For this review, use the dimensioned drawing (mm, ordinates from the lowest corner) and the shaded views. A direction names the side the tool comes from. Round coordinates to 2 decimals unless told otherwise and drop trailing zeros. Write each loop counter-clockwise with the first axis right and the second up, starting at its lowest first coordinate (ties: lowest second). Pieces come first, ordered by that corner, then holes. Notation, with made-up numbers: M -16.75,27.25 L 31.25,27.25 A19 cw 31.25,36.25 Z; hole C 76,-1.5 d7. An arc over 180 degrees is marked long. Use one line per item in the form item = value. Start each with the question number.
Item 1: Add section B-B (z = 2). State the section outline as (x, y) points.
Item 2: For the marked faces 1, 2, 3, 4 and 5, list the 3-axis set-ups (+Z, -Z, +X, -X, +Y, -Y) from which the entire face can be reached by the end or side of a thin tool; tool diameter is ignored.
Item 3: Draft analysis for pull direction X (two halves, no side actions). For the marked faces 6, 7 and 8, state which applies: released by +X, released by -X, zero draft, split by the parting line, or undercut.
Item 4: For P1, Ø1.2, axis at y = 12, z = 5, coming from the -X side; P2, Ø2, axis at x = 5.5, z = 4, coming from the +Y side; P3, Ø4, axis at x = 1.5, z = 5, coming from the -Y side; P4, Ø3, axis at y = 2.5, z = 6.5, coming from the +X side, all flat-tipped, find the tip position at first contact; note any pin that passes through.
Item 5: Add section D-D (z = 4.25). Count the separate pieces of the cut face and the enclosed holes in it, and give its area (3 significant figures).
Item 6: For line 1 (X direction, y = 13.25, z = 5); line 2 (Y direction, x = 5, z = 3.6); line 3 (Z direction, x = 1.95, y = 12), list the stretches that pass through material, from the lowest coordinate up. Write a range as [from, to].
Item 7: Add section A-A (y = 9.5). State the section outline as (x, z) points, and give its area (3 significant figures).
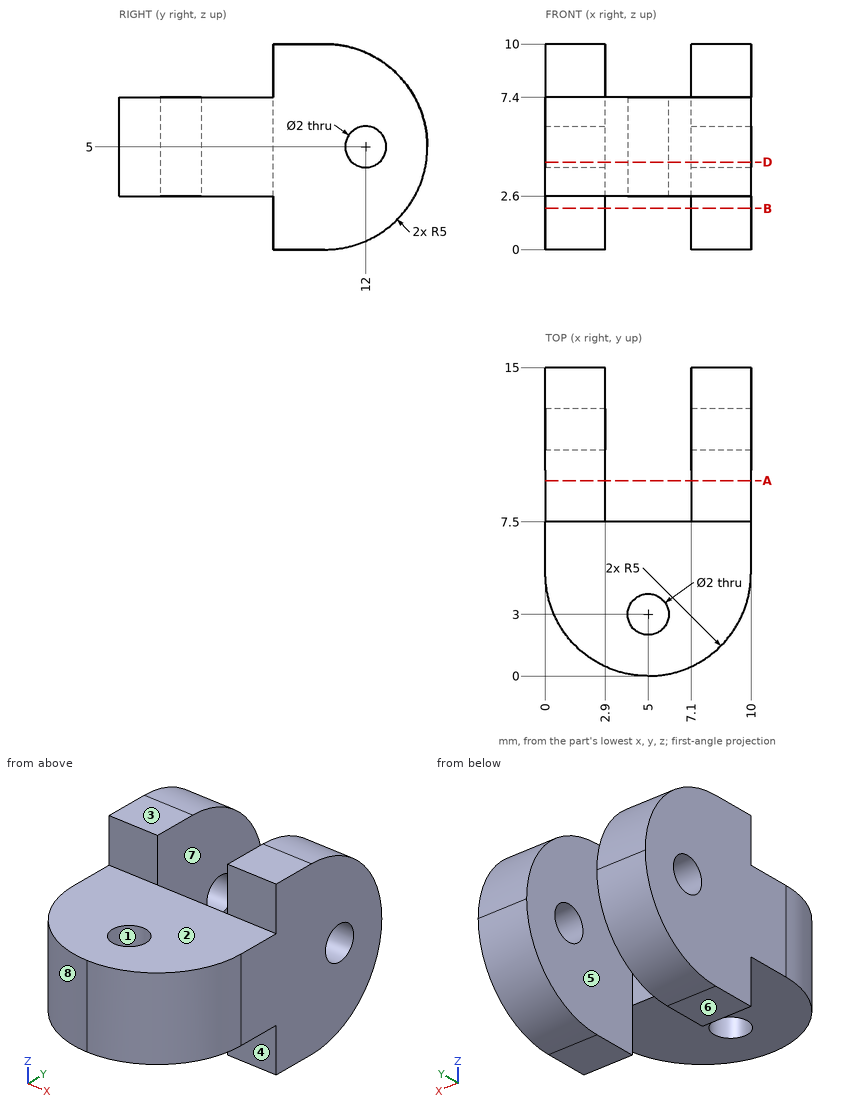
Calculated:
q1.outline = M 0,7.5 L 2.9,7.5 L 2.9,14 L 0,14 Z; M 7.1,7.5 L 10,7.5 L 10,14 L 7.1,14 Z
q2.face_1 = +Z, -Z
q2.face_2 = +Z, +X, -X, -Y
q2.face_3 = +Z, +X, -X, +Y, -Y
q2.face_4 = -Z, +X, -X, -Y
q2.face_5 = +Z, -Z, +Y
q3.face_6 = zero draft
q3.face_7 = undercut
q3.face_8 = released by -X
q4.P1 = through
q4.P2 = 7.5
q4.P3 = 0.23
q4.P4 = 9.9
q5.separate_pieces = 3
q5.enclosed_holes = 1
q5.area = 96.6 mm^2
q6.line_1 = [0, 2.9], [7.1, 10]
q6.line_2 = [0, 2], [4, 7.5]
q6.line_3 = [0.42, 4], [6, 9.58]
q7.outline = M 0,0 L 2.9,0 L 2.9,10 L 0,10 Z; M 7.1,0 L 10,0 L 10,10 L 7.1,10 Z
q7.area = 58.0 mm^2
